Verification items for the finished model (mm, model axes). A direction names the side the tool comes from. Coordinates: 2 decimals unless noted, no trailing zeros. Write each loop counter-clockwise with the first axis right and the second up, starting at its lowest first coordinate (ties: lowest second). Pieces come first, ordered by that corner, then holes. Notation, with made-up numbers: (0.25, -2.75) -> (33.25, -2.75) arc R26 ccw to (33.25, 28.25) -> close; hole circle Ø2 at (40, 30). An arc over 180 degrees is marked (long way). Answer in a Markdown table with one row per item.
```python
from build123d import *

# Parameters (mm, degrees)
F1_DEPTH = 1.5
F2_W     = 100.99
F2_H     = 60.99
F3_DEPTH = 3
F4_W     = 98
F4_H     = 58
F5_DEPTH = 3
F6_DEPTH = 25


with BuildPart() as f1:
    # F0 (on Top) → F1 (new body)
    with BuildSketch(Plane.XY):
        Polygon((-52.5, -32.5), (52.5, -32.5), (52.5, 32.5), (-39.427131, 32.5), (-52.5, 15.85602), align=None)
        Polygon((-52.5, 32.5), (-52.5, 15.85602), (-39.427131, 32.5), align=None)
    extrude(amount=F1_DEPTH)

    # F2 (on face) → F3 (join)
    with BuildSketch(Plane.XY.offset(1.5)):
        Rectangle(F2_W, F2_H)
    extrude(amount=F3_DEPTH)

    # F4 (on face) → F5 (cut)
    with BuildSketch(Plane.XY.offset(4.5)):
        Rectangle(F4_W, F4_H)
    extrude(amount=-F5_DEPTH, mode=Mode.SUBTRACT)

    # F0 (on Top) → F6 (cut)
    with BuildSketch(Plane.XY):
        Polygon((-52.5, 32.5), (-52.5, 15.85602), (-39.427131, 32.5), align=None)
    extrude(amount=F6_DEPTH, mode=Mode.SUBTRACT)


solid = f1.part
```
1. Section check B-B, the plane y = -18. Record the boundary of the cut face in (x, z) (3 decimals).
Geometry says:
| item | result |
|---|---|
| outline | (-52.5, 0) -> (52.5, 0) -> (52.5, 1.5) -> (50.495, 1.5) -> (50.495, 4.5) -> (49, 4.5) -> (49, 1.5) -> (-49, 1.5) -> (-49, 4.5) -> (-50.495, 4.5) -> (-50.495, 1.5) -> (-52.5, 1.5) -> close |
2. Depth check by flat-ended pin: P1, Ø1, axis at y = 24, z = 0.5, coming from the -X side; P2, Ø1.5, axis at y = -16.5, z = 2.5, coming from the +X side (3 decimals); P3, Ø1, axis at y = 12, z = 2.5, coming from the -X side (3 decimals). Enter the tip coordinate at first touch or a pass-through.
Geometry says:
| item | result |
|---|---|
| P1 | x = -46.5 |
| P2 | x = 50.495 |
| P3 | x = -50.495 |
3. Section check A-A, the plane x = 26. Record the boundary of the cut face in (y, z) (3 decimals), plus the area to 3 significant figures.
Geometry says:
| item | result |
|---|---|
| outline | (-32.5, 0) -> (32.5, 0) -> (32.5, 1.5) -> (30.495, 1.5) -> (30.495, 4.5) -> (29, 4.5) -> (29, 1.5) -> (-29, 1.5) -> (-29, 4.5) -> (-30.495, 4.5) -> (-30.495, 1.5) -> (-32.5, 1.5) -> close |
| area | 106 mm^2 |
4. Section check C-C, the plane z = 3.05. Record the boundary of the cut face in (x, y) (3 decimals), plus the area to 3 significant figures.
Geometry says:
| item | result |
|---|---|
| outline | (-50.495, -30.495) -> (50.495, -30.495) -> (50.495, 30.495) -> (-41.002, 30.495) -> (-42.176, 29) -> (49, 29) -> (49, -29) -> (-49, -29) -> (-49, 20.312) -> (-50.495, 18.409) -> close |
| area | 448 mm^2 |
5. Tool access check on faces 1 (the flat face through (-1, 0, 1.5)), 2 (the flat face through (-50.495, -6, 3)), 3 (the flat face through (4, 30.495, 3)). Record the directions out of +Z, -Z, +X, -X, +Y, -Y that give a thin tool (end or side, any length) a straight path to the whole face; none if there is none.
Geometry says:
| item | result |
|---|---|
| face 1 | +Z |
| face 2 | +Z, -X, +Y, -Y |
| face 3 | +Z, +X, -X, +Y |
6. Section check D-D, the plane x = -44. Record the boundary of the cut face in (y, z) (3 decimals).
Geometry says:
| item | result |
|---|---|
| outline | (-32.5, 0) -> (26.678, 0) -> (26.678, 1.5) -> (-29, 1.5) -> (-29, 4.5) -> (-30.495, 4.5) -> (-30.495, 1.5) -> (-32.5, 1.5) -> close |
7. Thickness scan on line 1 (X direction, y = 10, z = 3.4) (3 decimals); line 2 (Y direction, x = 33, z = 1.7) (3 decimals); line 3 (Z direction, x = 43, y = -18). Record the ranges inside material, lowest first. Write a range as from..to.
Geometry says:
| item | result |
|---|---|
| line 1 | -50.495..-49, 49..50.495 |
| line 2 | -30.495..-29, 29..30.495 |
| line 3 | 0..1.5 |
8. Mould release check, pull along Y, two halves, no side actions. Record for faces 4 (the flat face through (-1, -29, 3)), 5 (the flat face through (49, 0, 3)), 6 (the flat face through (-46.055, 24.062, 1.219)), 7 (the flat face through (50.495, 0, 3)): released by +Y, released by -Y, zero draft, split by the parting line, or undercut.
Geometry says:
| item | result |
|---|---|
| face 4 | undercut |
| face 5 | undercut |
| face 6 | released by +Y |
| face 7 | zero draft |
